from build123d import *

# Parameters (mm, degrees)
SKETCH1_R           = 12.5
BOSS_EXTRUDE1_DEPTH = 93.6
SKETCH2_R           = 15
BOSS_EXTRUDE2_DEPTH = 56
SKETCH3_R           = 10
BOSS_EXTRUDE3_DEPTH = 45
SKETCH4_R           = 4.755
CUT_EXTRUDE1_DEPTH  = 60
FILLET2_R           = 2
FILLET3_R           = 1.5
FILLET4_R           = 2


with BuildPart() as part:
    # Sketch1 → Boss-Extrude1 (new body)
    with BuildSketch(Plane.XY):
        Circle(SKETCH1_R)
    extrude(amount=BOSS_EXTRUDE1_DEPTH)

    # Sketch2 → Boss-Extrude2 (add)
    with BuildSketch(Plane.XY.offset(76)):
        Circle(SKETCH2_R)
    extrude(amount=-BOSS_EXTRUDE2_DEPTH)

    # Sketch3 → Boss-Extrude3 (add)
    with BuildSketch(Plane(origin=(0, 0, 0), x_dir=(-1, 0, 0), z_dir=(0, 0, -1))):
        Circle(SKETCH3_R)
    extrude(amount=BOSS_EXTRUDE3_DEPTH)

    # Sketch4 → Cut-Extrude1 (cut)
    with BuildSketch(Plane.XY.offset(93.6)):
        Circle(SKETCH4_R)
    extrude(amount=-CUT_EXTRUDE1_DEPTH, mode=Mode.SUBTRACT)

    # Fillet2
    fillet2_edges = [part.edges().sort_by_distance(p)[0] for p in [
        (-12.5, 0, 76),
    ]]
    fillet(fillet2_edges, radius=FILLET2_R)

    # Fillet3
    fillet3_edges = [part.edges().sort_by_distance(p)[0] for p in [
        (-12.5, 0, 20),
    ]]
    fillet(fillet3_edges, radius=FILLET3_R)

    # Fillet4
    fillet4_edges = [part.edges().sort_by_distance(p)[0] for p in [
        (10, 0, 0),
    ]]
    fillet(fillet4_edges, radius=FILLET4_R)


solid = part.part
The model under review builds one solid part; all positions refer to its coordinate system, in mm. A direction names the side the tool comes from. Round coordinates to 2 decimals unless told otherwise and drop trailing zeros. Write each loop counter-clockwise with the first axis right and the second up, starting at its lowest first coordinate (ties: lowest second). Pieces come first, ordered by that corner, then holes. Notation, with made-up numbers: (28.25, -15.5) - (70.25, -15.5) arc R26 cw to (70.25, 13.5) - close; hole circle Ø9 at (39.25, 25). An arc over 180 degrees is marked (long way). One line per item, written item: value. Start each with the question number.
1. The part is to be moulded in two halves that separate along Y. For faces 4 (the face through (4.535, 1.428, 64.02)), 5 (the face through (0, 0, -45)), 6 (the face through (0, 0, 33.6)), 7 (the face through (-14.985, 0.66, 48.392)), say which applies: released by +Y, released by -Y, zero draft, split by the parting line, or undercut.
2. Consider section D-D on z = 74. Write out the cut boundary in (x, y) (3 decimals), and give its area (3 significant figures).
3. Consider section A-A on x = 0. Write out the cut boundary in (y, z) (3 decimals), and give its area (3 significant figures).
4. Consider section C-C on z = 28.5. Write out the cut boundary in (x, y), and give its area (3 significant figures).
5. Machinability: for faces 1 (the face through (0, -5, 93.6)), 2 (the face through (2.17, -9.76, -23.2)), 3 (the face through (11.923, 3.755, 85.691)), which of the approach directions +Z, -Z, +X, -X, +Y, -Y give a long, thin tool a straight path to every point of the face, cutting with its end or side? Answer none if there is none.
6. To check wall thickness, follow L1, parallel to Y at x = 0, z = 58.5 (3 decimals); L2, parallel to Z at x = -2.25, y = -2; L3, parallel to Z at x = -1.25, y = 11.5. State the ranges of each line that lie inside material, in increasing order. Write a range as from..to.
7. Clearance check with flat-ended pins moving along their axes: P1, Ø3, axis at y = -3.5, z = 53.5, coming from the -X side; P2, Ø3, axis at x = 8.5, z = 11, coming from the +Y side; P3, Ø1.5, axis at x = 11.5, z = 75, coming from the -Y side; P4, Ø5, axis at x = -2.5, y = 1.5, coming from the +Z side. State where each tip first meets the part, or that it passes through.
Checks:
1. face 4: undercut
1. face 5: zero draft
1. face 6: undercut
1. face 7: split by the parting line
2. outline: circle Ø30 at (0, 0); hole circle Ø9.51 at (0, 0)
2. area: 636 mm^2
3. outline: (-15, 20) - (-14, 20) arc R1.5 cw to (-12.5, 18.5) - (-12.5, 0) - (-12, 0) arc R2 cw to (-10, -2) - (-10, -45) - (10, -45) - (10, -2) arc R2 cw to (12, 0) - (12.5, 0) - (12.5, 18.5) arc R1.5 cw to (14, 20) - (15, 20) - (15, 76) - (14.5, 76) arc R2 cw to (12.5, 78) - (12.5, 93.6) - (4.755, 93.6) - (4.755, 33.6) - (-4.755, 33.6) - (-4.755, 93.6) - (-12.5, 93.6) - (-12.5, 78) arc R2 cw to (-14.5, 76) - (-15, 76) - close
3. area: 2,950 mm^2
4. outline: circle Ø30 at (0, 0)
4. area: 707 mm^2
5. face 1: +Z, +X, -X, +Y, -Y
5. face 2: -Z
5. face 3: +Z
6. L1: y = -15..-4.755, 4.755..15
6. L2: z = -45..33.6
6. L3: z = -0.05..93.6
7. P1: stops at x = -14.87
7. P2: stops at y = 10.36
7. P3: stops at y = -10.46
7. P4: stops at z = 93.6
